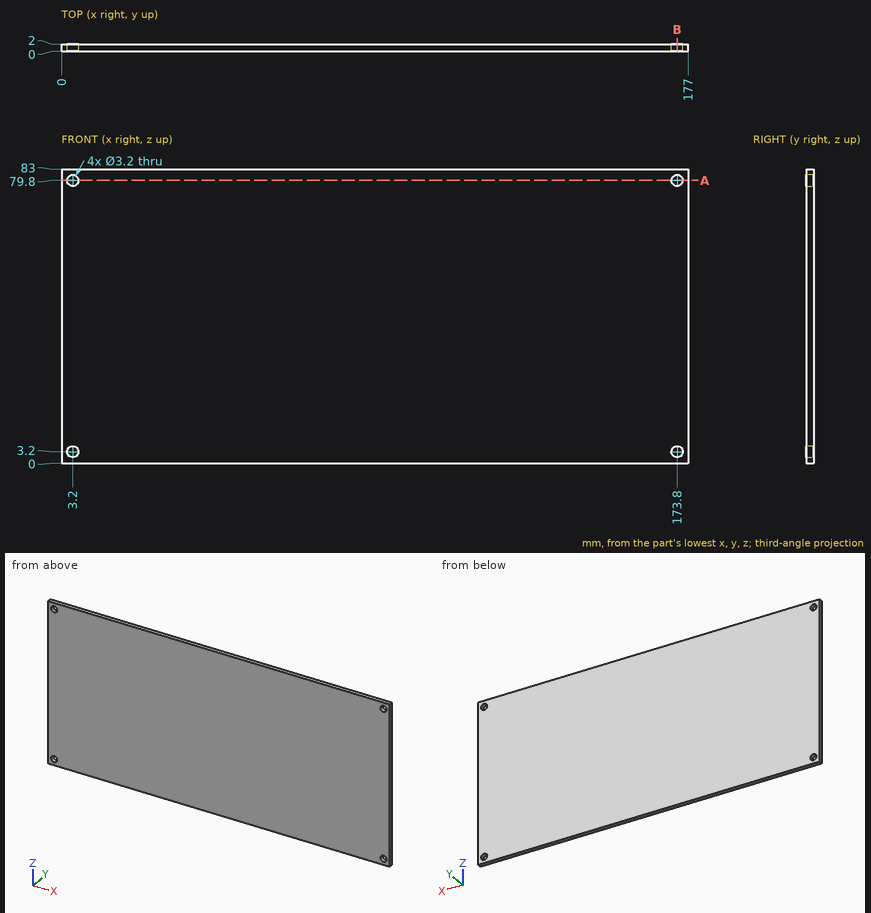
The drawing under review shows one solid part. Ordinate dimensions are in mm from its lowest x, y, z. Coordinates: 2 decimals unless noted, no trailing zeros. Loops run counter-clockwise (first coordinate to the right, second up) from the corner with the lowest first, then second, coordinate; pieces in that order, holes last. Notation, with made-up numbers: (40, 78.25) -> (76, 78.25) arc R17 cw to (76, 98.25) -> close; hole circle Ø4 at (38.5, 32.5). An arc over 180 degrees is marked (long way). Answer as a JSON object with one key per item and string values.
Q1. To check wall thickness, follow L1, parallel to X at y = 1.25, z = 3.2; L2, parallel to Z at x = 173.8, y = 1.1. State the ranges of each line that lie inside material, in increasing order.
Answer block:
{"L1": "x = 0 to 1.6, 4.8 to 172.2, 175.4 to 177", "L2": "z = 0 to 1.6, 4.8 to 78.2, 81.4 to 83"}
Q2. Take a section at B-B on x = 173.8. Give the boundary of the cut face in (y, z), plus the area to 3 significant figures.
Answer block:
{"outline": "(0, 0) -> (2, 0) -> (2, 1.6) -> (0, 1.6) -> close; (0, 4.8) -> (2, 4.8) -> (2, 78.2) -> (0, 78.2) -> close; (0, 81.4) -> (2, 81.4) -> (2, 83) -> (0, 83) -> close", "area": "153 mm^2"}
Q3. Clearance check with a flat-ended pin moving along its axis: pin 1 Ø4 at (x, z) = (21, 51.5) entering from -Y. State where the tip first meets the part, or that it passes through.
Answer block:
{"pin 1": "stops at y = 0"}
Q4. Take a section at A-A on z = 79.8. Give the boundary of the cut face in (x, y), plus the area to 3 significant figures.
Answer block:
{"outline": "(0, 0) -> (1.6, 0) -> (1.6, 2) -> (0, 2) -> close; (4.8, 0) -> (172.2, 0) -> (172.2, 2) -> (4.8, 2) -> close; (175.4, 0) -> (177, 0) -> (177, 2) -> (175.4, 2) -> close", "area": "341 mm^2"}
